```python
from build123d import *

# Parameters (mm, degrees)
SKETCH1_R           = 20
BOSS_EXTRUDE1_DEPTH = 60
SKETCH2_R           = 22.5
BOSS_EXTRUDE2_DEPTH = 10
CUT_EXTRUDE1_DEPTH  = 8


with BuildPart() as part:
    # Sketch1 → Boss-Extrude1 (new body)
    with BuildSketch(Plane.XY):
        Circle(SKETCH1_R)
    extrude(amount=BOSS_EXTRUDE1_DEPTH)

    # Sketch2 → Boss-Extrude2 (add)
    with BuildSketch(Plane.XY.offset(60)):
        Circle(SKETCH2_R)
    extrude(amount=BOSS_EXTRUDE2_DEPTH)

    # Sketch3 → Cut-Extrude1 (cut)
    with BuildSketch(Plane.XY.offset(70)):
        Polygon((-20.207259422, 0), (-10.103629711, -17.5), (10.103629711, -17.5), (20.207259422, 0), (10.103629711, 17.5), (-10.103629711, 17.5), align=None)
    extrude(amount=-CUT_EXTRUDE1_DEPTH, mode=Mode.SUBTRACT)


solid = part.part
```
Verification items for the finished model (mm, model axes). A direction names the side the tool comes from. Round coordinates to 2 decimals unless told otherwise and drop trailing zeros. Order: outer loops, then holes, each group sorted by start corner. A loop starts at its lowest first (then second) coordinate and runs counter-clockwise, first axis right, second up.
1) Cross-section at B-B, the plane y = -3. Record the cut outline in (x, z), plus the area to 3 significant figures.
Geometry says:
outline: (-22.3, 60) - (-19.77, 60) - (-19.77, 0) - (19.77, 0) - (19.77, 60) - (22.3, 60) - (22.3, 70) - (18.48, 70) - (18.48, 62) - (-18.48, 62) - (-18.48, 70) - (-22.3, 70) - close
area: 2,520 mm2
2) Tool access check on faces 1 (the cylindrical face through (10.382, -19.961, 64.93)), 2 (the flat face through (0, 17.5, 66)), 3 (the flat face through (-20.1, -1.6, 60)). Record the directions out of +Z, -Z, +X, -X, +Y, -Y that give a thin tool (end or side, any length) a straight path to the whole face; none if there is none.
Geometry says:
face 1: +Z, -Z
face 2: +Z
face 3: -Z
3) Cross-section at C-C, the plane z = 12.5. Record the cut outline in (x, y), plus the area to 3 significant figures.
Geometry says:
outline: circle Ø40 at (0, 0)
area: 1,260 mm2
4) Material ranges on line 1 (Z direction, x = 8.5, y = 8); line 2 (Z direction, x = -15, y = 16); line 3 (Y direction, x = 15, z = 19.5), recorded low to high.
Geometry says:
line 1: z = 0 to 62
line 2: z = 60 to 70
line 3: y = -13.23 to 13.23
5) Depth check by flat-ended pin: pin 1 (2.5 mm diameter, centred on x = -3, z = 65.5, fed in from +Y); pin 2 (2 mm diameter, centred on x = 3.5, z = 46, fed in from +Y); pin 3 (5 mm diameter, centred on y = 13.5, z = 12.5, fed in from +X). Enter the tip coordinate at first touch or a pass-through.
Geometry says:
pin 1: stops at y = 22.43
pin 2: stops at y = 19.84
pin 3: stops at x = 16.7
6) Draft check along Y on faces 4 (the flat face through (-15.226, -8.628, 66.056)), 5 (the flat face through (0, -17.5, 66)), 6 (the cylindrical face through (-4.336, -19.524, 29.58)), 7 (the flat face through (0, 0, 0)). Enter one of: +Y half, -Y half, draft (parallel to the pull), parting line (faces both ways), or undercut.
Geometry says:
face 4: undercut
face 5: undercut
face 6: parting line
face 7: draft
7) Cross-section at A-A, the plane x = 0. Record the cut outline in (y, z), plus the area to 3 significant figures.
Geometry says:
outline: (-22.5, 60) - (-20, 60) - (-20, 0) - (20, 0) - (20, 60) - (22.5, 60) - (22.5, 70) - (17.5, 70) - (17.5, 62) - (-17.5, 62) - (-17.5, 70) - (-22.5, 70) - close
area: 2,570 mm2
